from build123d import *

# Parameters (mm, degrees)
SKETCH1_R                                       = 25
BOSS_EXTRUDE1_DEPTH                             = 4
SKETCH2_R                                       = 16.5
BOSS_EXTRUDE2_DEPTH                             = 10
SKETCH3_R                                       = 12.5
CUT_EXTRUDE1_DEPTH                              = 11.5
SKETCH4_R                                       = 4
CUT_EXTRUDE2_DEPTH                              = 4
M3_CLEARANCE_HOLE1_D                            = 3.4
M3_CLEARANCE_HOLE1_DEPTH                        = 10
CSK_FOR_M3_FLAT_HEAD_MACHINE_SCREW1_D           = 3.4
CSK_FOR_M3_FLAT_HEAD_MACHINE_SCREW1_CSINK_D     = 6.3
CSK_FOR_M3_FLAT_HEAD_MACHINE_SCREW1_CSINK_ANGLE = 90
CIRPATTERN1_COUNT                               = 4
SKETCH10_R                                      = 13.125
CUT_EXTRUDE3_DEPTH                              = 11.5
CUT_EXTRUDE4_DEPTH                              = 10


with BuildPart() as part:
    # Sketch1 → Boss-Extrude1 (new body)
    with BuildSketch(Plane(origin=(0, 0, 0), x_dir=(0, 0, -1), z_dir=(1, 0, 0))):
        Circle(SKETCH1_R)
    extrude(amount=BOSS_EXTRUDE1_DEPTH)

    # Sketch2 → Boss-Extrude2 (add)
    with BuildSketch(Plane(origin=(4, 0, 0), x_dir=(0, 0, -1), z_dir=(1, 0, 0))):
        Circle(SKETCH2_R)
    extrude(amount=BOSS_EXTRUDE2_DEPTH)

    # Sketch3 → Cut-Extrude1 (cut)
    with BuildSketch(Plane.ZY):
        Circle(SKETCH3_R)
    extrude(amount=-CUT_EXTRUDE1_DEPTH, mode=Mode.SUBTRACT)

    # Sketch4 → Cut-Extrude2 (cut)
    with BuildSketch(Plane(origin=(14, 0, 0), x_dir=(0, 0, -1), z_dir=(1, 0, 0))):
        Circle(SKETCH4_R)
    extrude(amount=-CUT_EXTRUDE2_DEPTH, mode=Mode.SUBTRACT)

    # M3 Clearance Hole1
    with Locations(Plane(origin=(14, 0, 0), x_dir=(0, 0, -1), z_dir=(1, 0, 0))):
        with Locations((8.5, 0), (-8.5, 0)):
            Hole(M3_CLEARANCE_HOLE1_D / 2, depth=M3_CLEARANCE_HOLE1_DEPTH)

    # CSK for M3 Flat Head Machine Screw1 (through all)
    with Locations(Plane(origin=(4, 0, 0), x_dir=(0, 0, -1), z_dir=(1, 0, 0))):
        with Locations((-14.495689014, -14.495689014)):
            csk_for_m3_flat_head_machine_screw1 = CounterSinkHole(CSK_FOR_M3_FLAT_HEAD_MACHINE_SCREW1_D / 2, CSK_FOR_M3_FLAT_HEAD_MACHINE_SCREW1_CSINK_D / 2, counter_sink_angle=CSK_FOR_M3_FLAT_HEAD_MACHINE_SCREW1_CSINK_ANGLE)

    # CirPattern1: CSK for M3 Flat Head Machine Screw1 ×4 about axis
    cirpattern1_axis = Axis((0, 0, 0), (1, 0, 0))
    for i in range(1, CIRPATTERN1_COUNT):
        add(csk_for_m3_flat_head_machine_screw1.rotate(cirpattern1_axis, i * 360 / CIRPATTERN1_COUNT), mode=Mode.SUBTRACT)

    # Sketch10 → Cut-Extrude3 (cut)
    with BuildSketch(Plane.ZY):
        Circle(SKETCH10_R)
    extrude(amount=-CUT_EXTRUDE3_DEPTH, mode=Mode.SUBTRACT)

    # Sketch12 → Cut-Extrude4 (cut)
    with BuildSketch(Plane(origin=(4, 0, 0), x_dir=(0, 0, -1), z_dir=(1, 0, 0))):
        with BuildLine():
            Line((-4, 20.75), (-4, 23.473389189))
            ThreePointArc((-4, 23.473389189), (-4.37084713, 24.250670776), (-5.208333333, 24.451447071))
            ThreePointArc((-5.208333333, 24.451447071), (0, 25), (5.208333333, 24.451447071))
            ThreePointArc((5.208333333, 24.451447071), (4.37084713, 24.250670776), (4, 23.473389189))
            Line((4, 23.473389189), (4, 20.75))
            ThreePointArc((4, 20.75), (0, 16.75), (-4, 20.75))
        make_face()
        with BuildLine():
            Line((4, -20.75), (4, -23.473389189))
            ThreePointArc((4, -23.473389189), (4.37084713, -24.250670776), (5.208333333, -24.451447071))
            ThreePointArc((5.208333333, -24.451447071), (0, -25), (-5.208333333, -24.451447071))
            ThreePointArc((-5.208333333, -24.451447071), (-4.37084713, -24.250670776), (-4, -23.473389189))
            Line((-4, -23.473389189), (-4, -20.75))
            ThreePointArc((-4, -20.75), (0, -16.75), (4, -20.75))
        make_face()
    extrude(amount=-CUT_EXTRUDE4_DEPTH, mode=Mode.SUBTRACT)


solid = part.part
Geometry check sheet. Reference: the model listing, model coordinates, mm. A direction names the side the tool comes from. Round coordinates to 2 decimals unless told otherwise and drop trailing zeros. Write each loop counter-clockwise with the first axis right and the second up, starting at its lowest first coordinate (ties: lowest second). Pieces come first, ordered by that corner, then holes.
Item 1: Section check B-B (y = 0). Record the boundary of the cut face in (x, z) (3 decimals).
Determined:
outline: (0, -25) - (4, -25) - (4, -16.5) - (14, -16.5) - (14, -10.2) - (11.5, -10.2) - (11.5, -13.125) - (0, -13.125) - close; (0, 13.125) - (11.5, 13.125) - (11.5, 10.2) - (14, 10.2) - (14, 16.5) - (4, 16.5) - (4, 25) - (0, 25) - close; (11.5, -6.8) - (14, -6.8) - (14, -4) - (11.5, -4) - close; (11.5, 4) - (14, 4) - (14, 6.8) - (11.5, 6.8) - close
Item 2: Go/stop test with flat-tipped pins: pin 1 Ø6 at (x, z) = (5.5, -2) entering from -Y; pin 2 Ø9 at (y, z) = (0, 0) entering from -X; pin 3 Ø0.8 at (x, y) = (1.5, -21.5) entering from +Z. Record where each tip stops, or that it passes through.
Determined:
pin 1: stops at y = -24.39
pin 2: stops at x = 11.5
pin 3: stops at z = 13.41
Item 3: Section check D-D (x = 1.5). Record the boundary of the cut face in (y, z) (3 decimals), plus the area to 3 significant figures.
Determined:
outline: (-24.451, -5.208) arc R25 ccw to (24.451, -5.208) arc R1 ccw to (23.473, -4) - (20.75, -4) arc R4 cw to (20.75, 4) - (23.473, 4) arc R1 ccw to (24.451, 5.208) arc R25 ccw to (-24.451, 5.208) arc R1 ccw to (-23.473, 4) - (-20.75, 4) arc R4 cw to (-20.75, -4) - (-23.473, -4) arc R1 ccw to start; hole circle Ø3.4 at (-14.496, -14.496); hole circle Ø3.4 at (-14.496, 14.496); hole circle Ø26.25 at (0, 0); hole circle Ø3.4 at (14.496, -14.496); hole circle Ø3.4 at (14.496, 14.496)
area: 1,270 mm2
Item 4: Section check A-A (z = 0). Record the boundary of the cut face in (x, y) (3 decimals), plus the area to 3 significant figures.
Determined:
outline: (0, -16.75) - (4, -16.75) - (4, -16.5) - (14, -16.5) - (14, -4) - (11.5, -4) - (11.5, -13.125) - (0, -13.125) - close; (0, 13.125) - (11.5, 13.125) - (11.5, 4) - (14, 4) - (14, 16.5) - (4, 16.5) - (4, 16.75) - (0, 16.75) - close
area: 142 mm2
Item 5: Mould release check, pull along Y, two halves, no side actions. Record for faces 4 (the face through (1.26, -13.24, -13.35)), 5 (the face through (2, 22, -4)), 6 (the face through (8.93, -6.32, -15.24)): +Y half, -Y half, draft (parallel to the pull), parting line (faces both ways), or undercut.
Determined:
face 4: undercut
face 5: draft
face 6: parting line
Item 6: Material ranges on line 1 along Y through (x, z) = (13.45, 0); line 2 along Y through (x, z) = (11.25, 0) (3 decimals); line 3 along X through (y, z) = (-12, 0), recorded low to high.
Determined:
line 1: y = -16.5 to -4, 4 to 16.5
line 2: y = -16.5 to -13.125, 13.125 to 16.5
line 3: x = 11.5 to 14
Item 7: Access from +Z, -Z, +X, -X, +Y, -Y to the whole of each face (thin tool, end or side, straight path). Record for faces 1 (the face through (2, -22, 4)), 2 (the face through (11.5, -3, -3)), 3 (the face through (2, 22, 4)).
Determined:
face 1: +X, -X, -Y
face 2: -X
face 3: +X, -X, +Y
Item 8: Section check C-C (y = 19). Record the boundary of the cut face in (x, z), plus the area to 3 significant figures.
Determined:
outline: (0, -16.25) - (4, -16.25) - (4, -3.6) - (0, -3.6) - close; (0, 3.6) - (4, 3.6) - (4, 16.25) - (0, 16.25) - close
area: 101 mm2
